Part model, mm, in its own coordinate system. Face numbers are marked on the shaded views. A direction names the side the tool comes from. Coordinates: 2 decimals unless noted, no trailing zeros. Write each loop counter-clockwise with the first axis right and the second up, starting at its lowest first coordinate (ties: lowest second). Pieces come first, ordered by that corner, then holes. Notation, with made-up numbers: (62, 68.25) - (93, 68.25) arc R22 cw to (93, 97.25) - close; hole circle Ø1 at (63, 49). An arc over 180 degrees is marked (long way). Use a Markdown table: item, result.
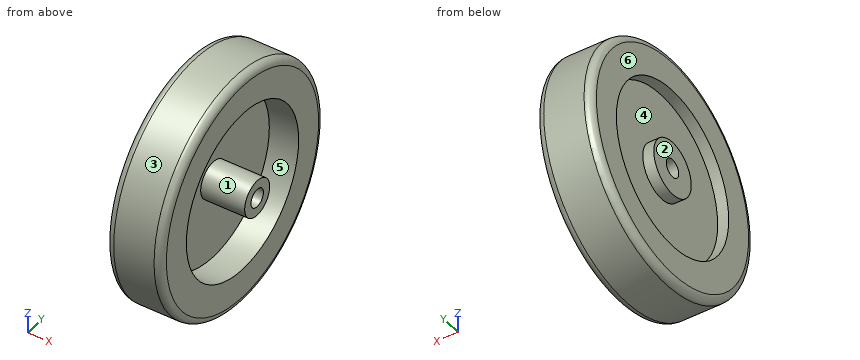
```python
from build123d import *

# Parameters (mm, degrees)
SKETCH_R        = 32.5
SKETCH_R_2      = 2.5
PAD_DEPTH       = 15
SKETCH001_R     = 5
SKETCH001_R_2   = 2.5
PAD001_DEPTH    = 4
SKETCH002_R     = 22.5
SKETCH002_R_2   = 7.5
POCKET_DEPTH    = 3
SKETCH003_R     = 22.5
SKETCH003_R_2   = 5
POCKET001_DEPTH = 8
FILLET_R        = 2
FILLET001_R     = 2


with BuildPart() as part:
    # Sketch → Pad (new body)
    with BuildSketch(Plane.YZ):
        Circle(SKETCH_R)
        Circle(SKETCH_R_2, mode=Mode.SUBTRACT)
    extrude(amount=PAD_DEPTH)

    # Sketch001 (on Face4 of Pad) → Pad001 (join)
    with BuildSketch(Plane.YZ.offset(15)):
        Circle(SKETCH001_R)
        Circle(SKETCH001_R_2, mode=Mode.SUBTRACT)
    extrude(amount=PAD001_DEPTH)

    # Sketch002 (on Face2 of Pad001) → Pocket (cut)
    with BuildSketch(Plane(origin=(0, 0, 0), x_dir=(0, 1, 0), z_dir=(-1, 0, 0))):
        Circle(SKETCH002_R)
        Circle(SKETCH002_R_2, mode=Mode.SUBTRACT)
    extrude(amount=-POCKET_DEPTH, mode=Mode.SUBTRACT)

    # Sketch003 (on Face3 of Pocket) → Pocket001 (cut)
    with BuildSketch(Plane.YZ.offset(15)):
        Circle(SKETCH003_R)
        Circle(SKETCH003_R_2, mode=Mode.SUBTRACT)
    extrude(amount=-POCKET001_DEPTH, mode=Mode.SUBTRACT)

    # Fillet
    fillet_edges = [part.edges().sort_by_distance(p)[0] for p in [
        (15, -32.5, 0),
    ]]
    fillet(fillet_edges, radius=FILLET_R)

    # Fillet001
    fillet001_edges = [part.edges().sort_by_distance(p)[0] for p in [
        (0, -32.5, 0),
    ]]
    fillet(fillet001_edges, radius=FILLET001_R)


solid = part.part
```
Item 1: Drop flat-ended pins along their axis: P1, Ø5, axis at x = 6, z = -24, coming from the +Y side; P2, Ø4.5, axis at y = 0, z = 0, coming from the +X side; P3, Ø1, axis at y = -4, z = 11, coming from the -X side; P4, Ø6, axis at x = 6.5, y = 17, coming from the -Z side. Give the stop position or say it passes through.
From the geometry:
| item | result |
|---|---|
| P1 | y = 24.37 |
| P2 | through |
| P3 | x = 3 |
| P4 | z = -29.33 |
Item 2: Band-saw the part on A-A, the plane y = 0. Give the cut face in (x, z), then the cut area to 3 significant figures.
From the geometry:
| item | result |
|---|---|
| outline | (0, -30.5) arc R2 ccw to (2, -32.5) - (13, -32.5) arc R2 ccw to (15, -30.5) - (15, -22.5) - (7, -22.5) - (7, -5) - (19, -5) - (19, -2.5) - (0, -2.5) - (0, -7.5) - (3, -7.5) - (3, -22.5) - (0, -22.5) - close; (0, 2.5) - (19, 2.5) - (19, 5) - (7, 5) - (7, 22.5) - (15, 22.5) - (15, 30.5) arc R2 ccw to (13, 32.5) - (2, 32.5) arc R2 ccw to (0, 30.5) - (0, 22.5) - (3, 22.5) - (3, 7.5) - (0, 7.5) - close |
| area | 547 mm^2 |
Item 3: Band-saw the part on D-D, the plane x = 11.25. Give the cut face in (y, z), then the cut area to 3 significant figures.
From the geometry:
| item | result |
|---|---|
| outline | circle Ø65 at (0, 0); circle Ø10 at (0, 0); hole circle Ø45 at (0, 0); hole circle Ø5 at (0, 0) |
| area | 1,790 mm^2 |
Item 4: Which spindle directions (+Z, -Z, +X, -X, +Y, -Y) get a long thin tool onto all of the face, cutting with end or side? Do the marked faces 4, 5 and 6. Say none if no direction does.
From the geometry:
| item | result |
|---|---|
| face 4 | -X |
| face 5 | +X |
| face 6 | +Z, -Z, -X, +Y, -Y |
Item 5: Drill centre lines: probe 1 along Z at (x, y) = (1.9, 0); probe 2 along Z at (x, y) = (13, 0); probe 3 along Z at (x, y) = (5, 0). Where is each one in solid material? Low to high.
From the geometry:
| item | result |
|---|---|
| probe 1 | -32.5 to -22.5, -7.5 to -2.5, 2.5 to 7.5, 22.5 to 32.5 |
| probe 2 | -32.5 to -22.5, -5 to -2.5, 2.5 to 5, 22.5 to 32.5 |
| probe 3 | -32.5 to -2.5, 2.5 to 32.5 |
Item 6: Two-plate mould, pull along Z, no slides. Class the marked faces 1, 2 and 3: pulls with the +Z half, pulls with the -Z half, needs draft (parallel to the pull), parting line crosses it, or undercut.
From the geometry:
| item | result |
|---|---|
| face 1 | undercut |
| face 2 | needs draft |
| face 3 | parting line crosses it |
Item 7: Band-saw the part on C-C, the plane x = 16.25. Give the cut face in (y, z).
From the geometry:
| item | result |
|---|---|
| outline | circle Ø10 at (0, 0); hole circle Ø5 at (0, 0) |
